```python
from build123d import *

# Parameters (mm, degrees)
EXTRUDE_BODY_DEPTH = 10
SKETCH2_W          = 1.9
SKETCH2_H          = 0.9
CUT_EXTRUDE1_DEPTH = 11
SKETCH3_W          = 1.9
SKETCH3_H          = 0.9
CUT_EXTRUDE2_DEPTH = 11
CUT_EXTRUDE3_DEPTH = 11
HOLE_REVOLVE_D     = 3
EDGE_FILLETS_R     = 0.2


with BuildPart() as part:
    # Sketch1 → Extrude Body (new body)
    with BuildSketch(Plane.XY.offset(5)):
        Polygon((4.9, -1), (4.9, 0.9), (-4.9, 0.9), (-4.9, -1), (-2.3, -3.6), (2.3, -3.6), align=None)
    extrude(amount=-EXTRUDE_BODY_DEPTH)

    # Sketch2 → Cut-Extrude1 (cut, through all)
    with BuildSketch(Plane(origin=(0, 0, -5), x_dir=(-1, 0, 0), z_dir=(0, 0, -1))):
        with Locations((3.95, 0.45)):
            Rectangle(SKETCH2_W, SKETCH2_H)
    extrude(amount=-CUT_EXTRUDE1_DEPTH, mode=Mode.SUBTRACT)

    # Sketch3 → Cut-Extrude2 (cut, through all)
    with BuildSketch(Plane(origin=(0, 0, -5), x_dir=(-1, 0, 0), z_dir=(0, 0, -1))):
        with Locations((-3.95, 0.45)):
            Rectangle(SKETCH3_W, SKETCH3_H)
    extrude(amount=-CUT_EXTRUDE2_DEPTH, mode=Mode.SUBTRACT)

    # Sketch4 → Cut-Extrude3 (cut, through all)
    with BuildSketch(Plane(origin=(0, 0, -5), x_dir=(-1, 0, 0), z_dir=(0, 0, -1))):
        Polygon((0.4, 0.9), (-0.4, 0.9), (0, 0.5), align=None)
    extrude(amount=-CUT_EXTRUDE3_DEPTH, mode=Mode.SUBTRACT)

    # Hole Revolve (through all)
    with Locations(Plane(origin=(0, -3.6, 0), x_dir=(-1, 0, 0), z_dir=(0, -1, 0))):
        with Locations((0, 0)):
            Hole(HOLE_REVOLVE_D / 2)

    # Edge Fillets
    edge_fillets_edges = [part.edges().sort_by_distance(p)[0] for p in [
        (4.9, 0, 0),
        (3, 0, 0),
        (-4.9, -1, 0),
        (3, 0.9, 0),
        (-3, 0, 0),
        (0.4, 0.9, -3.222841615),
        (0, 0.5, 3.25),
        (-0.4, 0.9, -3.222841615),
        (4.9, -1, 0),
        (-3, 0.9, 0),
        (0, 0.5, -3.25),
        (-0.4, 0.9, 3.222841615),
        (-4.9, 0, 0),
        (-2.3, -3.6, 0),
        (0.4, 0.9, 3.222841615),
        (2.3, -3.6, 0),
    ]]
    fillet(edge_fillets_edges, radius=EDGE_FILLETS_R)


solid = part.part
```
Read the model definition and answer for the solid it produces. Units are mm, in the model's axes. A direction names the side the tool comes from. Give positions to 0.01 mm unless a question says otherwise; leave off trailing zeros. Order: outer loops, then holes, each group sorted by start corner. A loop starts at its lowest first (then second) coordinate and runs counter-clockwise, first axis right, second up.
(1) Find section A-A (z = 0). Give the vertices of the cut face in (x, y).
(2) For faces 5 (the flat face through (2, 0.9, 0)), 6 (the flat face through (4, 0, 0)), determine the directions among +Z, -Z, +X, -X, +Y, -Y from which every point of the face is accessible in a straight line to the end or side of a thin tool.
(3) Straight lines are drawn through the part: L1, parallel to Z at x = 0, y = -1.3; L2, parallel to Z at x = -1, y = 0.4; L3, parallel to Y at x = -2.25, z = 4.25. For each, find the intervals that lie inside material, in ascending order.
(4) Given pin 1 (1.6 mm diameter, centred on x = 4.5, z = -0.5, fed in from +Y), flat-ended and moving along its own axis, determine where the tip first touches the part or whether it passes through.
(5) Find section C-C (y = -1.5). Give the vertices of the cut face in (x, z).
(6) Find section B-B (x = 0). Give the vertices of the cut face in (y, z), plus the area to 3 significant figures.
(7) Find section D-D (z = -2.75). Give the vertices of the cut face in (x, y), plus the area to 3 significant figures.
(8) For a pull along X with two mould halves and no side action, classify faces 1 (the flat face through (-4, 0, 0)), 2 (the flat face through (-3.6, -2.3, 0.1)), 3 (the cylindrical face through (-1.5, -1.32, -0.07)), 4 (the flat face through (3.6, -2.3, 0.1)) as released by +X, released by -X, zero draft, split by the parting line, or undercut.
Result sheet:
1. outline: (-4.9, -0.92) arc R0.2 ccw to (-4.84, -1.06) - (-2.36, -3.54) arc R0.2 ccw to (-2.22, -3.6) - (-1.5, -3.6) - (-1.5, 0.9) - (-2.8, 0.9) arc R0.2 ccw to (-3, 0.7) - (-3, 0.2) arc R0.2 cw to (-3.2, 0) - (-4.7, 0) arc R0.2 ccw to (-4.9, -0.2) - close; (1.5, -3.6) - (2.22, -3.6) arc R0.2 ccw to (2.36, -3.54) - (4.84, -1.06) arc R0.2 ccw to (4.9, -0.92) - (4.9, -0.2) arc R0.2 ccw to (4.7, 0) - (3.2, 0) arc R0.2 cw to (3, 0.2) - (3, 0.7) arc R0.2 ccw to (2.8, 0.9) - (1.5, 0.9) - close
2. face 5: +Z, -Z, +X, -X, +Y
2. face 6: +Z, -Z, +X, +Y
3. L1: z = -5 to -1.5, 1.5 to 5
3. L2: z = -5 to -1.12, 1.12 to 5
3. L3: y = -3.6 to 0.9
4. pin 1: stops at y = 0
5. outline: (-4.4, -5) - (4.4, -5) - (4.4, 5) - (-4.4, 5) - close; hole circle Ø3 at (0, 0)
6. outline: (-3.6, -5) - (0.58, -5) - (0.58, -1.5) - (-3.6, -1.5) - close; (-3.6, 1.5) - (0.58, 1.5) - (0.58, 5) - (-3.6, 5) - close
6. area: 29.3 mm2
7. outline: (-4.9, -0.92) arc R0.2 ccw to (-4.84, -1.06) - (-2.36, -3.54) arc R0.2 ccw to (-2.22, -3.6) - (2.22, -3.6) arc R0.2 ccw to (2.36, -3.54) - (4.84, -1.06) arc R0.2 ccw to (4.9, -0.92) - (4.9, -0.2) arc R0.2 ccw to (4.7, 0) - (3.2, 0) arc R0.2 cw to (3, 0.2) - (3, 0.7) arc R0.2 ccw to (2.8, 0.9) - (0.48, 0.9) arc R0.2 ccw to (0.34, 0.84) - (0.14, 0.64) arc R0.2 cw to (-0.14, 0.64) - (-0.34, 0.84) arc R0.2 ccw to (-0.48, 0.9) - (-2.8, 0.9) arc R0.2 ccw to (-3, 0.7) - (-3, 0.2) arc R0.2 cw to (-3.2, 0) - (-4.7, 0) arc R0.2 ccw to (-4.9, -0.2) - close
7. area: 33.7 mm2
8. face 1: zero draft
8. face 2: released by -X
8. face 3: undercut
8. face 4: released by +X
